Geometry: see drawing. Coordinates: mm, zero at the bounding-box minimum. A direction names the side the tool comes from. Coordinates: 2 decimals unless noted, no trailing zeros. Write each loop counter-clockwise with the first axis right and the second up, starting at its lowest first coordinate (ties: lowest second). Pieces come first, ordered by that corner, then holes.
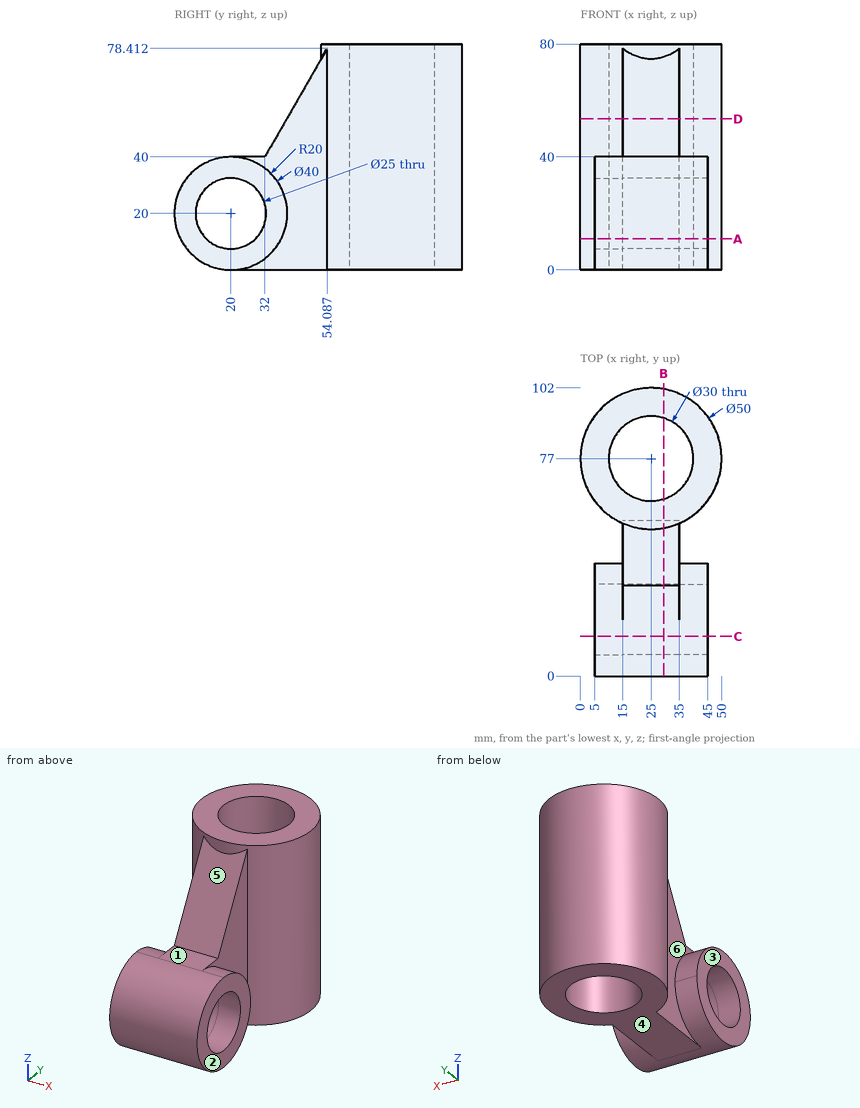
Item 1: Pull-direction query (Y, two-part tool) for the marked faces 4, 5 and 6; classes: released by +Y, released by -Y, zero draft, split by the parting line, or undercut.
Derived:
face 4: zero draft
face 5: released by -Y
face 6: undercut
Item 2: Section D-D, the plane z = 53.5. Output: boundary loops of the cut face in (x, y), plus the area to 4 significant figures.
Derived:
outline: (15, 39.76) - (35, 39.76) - (35, 54.09) arc R25 ccw (long way) to (15, 54.09) - close; hole circle Ø30 at (25, 77)
area: 1,515 mm2
Item 3: Section B-B, the plane x = 29.5. Output: boundary loops of the cut face in (y, z).
Derived:
outline: (20, 0) - (62.69, 0) - (62.69, 80) - (52.41, 80) - (52.41, 75.49) - (32, 40) - (20, 40) arc R20 ccw to start; (91.31, 0) - (101.59, 0) - (101.59, 80) - (91.31, 80) - close; hole circle Ø25 at (20, 20)
Item 4: Section C-C, the plane y = 14. Output: boundary loops of the cut face in (x, z), plus the area to 3 significant figures.
Derived:
outline: (5, 0.92) - (45, 0.92) - (45, 9.03) - (5, 9.03) - close; (5, 30.97) - (45, 30.97) - (45, 39.08) - (5, 39.08) - close
area: 649 mm2
Item 5: Pin query (flat end, axial travel): pin 1 (2 mm diameter, centred on x = 22, z = 49.5, fed in from +Y); pin 2 (8 mm diameter, centred on x = 19.5, y = 12.5, fed in from +Z); pin 3 (12 mm diameter, centred on y = 24.5, z = 19.5, fed in from +X); pin 4 (10 mm diameter, centred on x = 37, z = 36, fed in from +Y). Return the tip coordinate at first contact, or that it passes through.
Derived:
pin 1: stops at y = 101.92
pin 2: stops at z = 39.69
pin 3: passes through
pin 4: stops at y = 101
Item 6: Section A-A, the plane z = 11. Output: boundary loops of the cut face in (x, y) (1 decimal).
Derived:
outline: (5, 2.1) - (45, 2.1) - (45, 11.3) - (5, 11.3) - close; (5, 28.7) - (45, 28.7) - (45, 37.9) - (35, 37.9) - (35, 54.1) arc R25 ccw (long way) to (15, 54.1) - (15, 37.9) - (5, 37.9) - close; hole circle Ø30 at (25, 77)
Item 7: Material intervals for probe 1 along Z at (x, y) = (18.25, 20); probe 2 along Y at (x, z) = (37, 33); probe 3 along Y at (x, z) = (16, 8.5) (1 decimal), sorted ascending.
Derived:
probe 1: z = 0 to 7.5, 32.5 to 40
probe 2: y = 4.8 to 35.2, 55.07 to 68, 86 to 98.93
probe 3: y = 3.6 to 15.1, 24.9 to 65, 89 to 100.3
Item 8: Set-up query: the marked faces 1, 2 and 3. Return all of +Z, -Z, +X, -X, +Y, -Y with unobstructed straight access to the full face (end or side cutting, diameter ignored); none if empty.
Derived:
face 1: +Z, +X, -X, -Y
face 2: +Z, -Z, +X, -Y
face 3: +Z, -Z, -X, -Y
